Model file for the job. Use its own axes, mm. Give positions to 0.01 mm unless a question says otherwise; leave off trailing zeros. Order: outer loops, then holes, each group sorted by start corner. A loop starts at its lowest first (then second) coordinate and runs counter-clockwise, first axis right, second up. Notation, with made-up numbers: (3, 34) - (22, 34) arc R23 ccw to (22, 70) - close; hole circle Ø3 at (20.5, 45). An arc over 180 degrees is marked (long way). Return JSON: item names as keys, results as strings. Group by question number.
Autodesk Inventor part; units mm, degrees
ref_plane "YZ Plane" through (0, 0, 0) normal (1, 0, 0) x (0, 1, 0)
ref_plane "XZ Plane" through (0, 0, 0) normal (0, 1, 0) x (-1, 0, 0)
ref_plane "XY Plane" through (0, 0, 0) normal (0, 0, 1) x (1, 0, 0)
sketch "Sketch1" plane through (0, 0, 0) normal (0, 0, 1) x (1, 0, 0)
  line L0 (0, 0) -> (74.93, 0)
  line L1 (74.93, 0) -> (74.93, -46.99)
  line L2 (74.93, -46.99) -> (0, -46.99)
  line L3 (0, -46.99) -> (0, 0)
  dimension "d0" = 74.93
  dimension "d1" = 46.99
extrude "Extrusion1" add sketch "Sketch1" along normal blind 6.985
sketch "Sketch2" plane through (0, -46.99, 0) normal (0, -1, 0) x (1, 0, 0)
  line L0 (74.93, 6.985) -> (0, 6.985)
  circle A0 centre (33.02, 6.985) radius 3.175
  circle A1 centre (41.91, 6.985) radius 3.2056
  line L1 (74.93, 0) -> (74.93, 6.985)
  point P0 (0, 0)
  dimension "d4" = 6.35
  dimension "d5" = 8.89
  dimension "d6" = 33.02
extrude "Extrusion2" cut sketch "Sketch2" against normal blind 101.6
properties part number "Heatsink cu base" material "Copper"
(1) Drill centre lines: L1, parallel to X at y = -23.5, z = 5.5; L2, parallel to X at y = -14, z = 5.75; L3, parallel to Z at x = 41.5, y = -32. Where is each one in solid material? Low to high.
(2) Slice it at B-B (z = 6). Give the cut face in (x, y), and give its area (3 significant figures).
(3) Slice it at C-C (x = 41.91). Give the cut face in (y, z), and give its area (3 significant figures).
(4) Slice it at D-D (x = 33.02). Give the cut face in (y, z), and give its area (3 significant figures).
(5) Slice it at A-A (y = -28.5). Give the cut face in (x, z) (3 decimals), and give its area (3 significant figures).
Result set:
{
 "1": {"L1": "x = 0 to 30.21, 35.83 to 39.07, 44.75 to 74.93", "L2": "x = 0 to 30.1, 35.94 to 38.95, 44.87 to 74.93", "L3": "z = 0 to 3.81"},
 "2": {"outline": "(0, -46.99) - (30, -46.99) - (30, 0) - (0, 0) - close; (36.04, -46.99) - (38.86, -46.99) - (38.86, 0) - (36.04, 0) - close; (44.96, -46.99) - (74.93, -46.99) - (74.93, 0) - (44.96, 0) - close", "area": "2,950 mm²"},
 "3": {"outline": "(-46.99, 0) - (0, 0) - (0, 3.78) - (-46.99, 3.78) - close", "area": "178 mm²"},
 "4": {"outline": "(-46.99, 0) - (0, 0) - (0, 3.81) - (-46.99, 3.81) - close", "area": "179 mm²"},
 "5": {"outline": "(0, 0) - (74.93, 0) - (74.93, 6.985) - (45.116, 6.985) arc R3.206 cw to (38.704, 6.985) - (36.195, 6.985) arc R3.175 cw to (29.845, 6.985) - (0, 6.985) - close", "area": "491 mm²"}
}
